Source: CAD feature listing. Evaluate the final solid. Frame: model axes, mm. Face numbers are marked on the shaded views. A direction names the side the tool comes from. Round coordinates to 2 decimals unless told otherwise and drop trailing zeros. Loops run counter-clockwise (first coordinate to the right, second up) from the corner with the lowest first, then second, coordinate; pieces in that order, holes last. Notation, with made-up numbers: (62, -29.5) -> (111, -29.5) arc R16 cw to (111, -18.5) -> close; hole circle Ø11 at (55.25, -3). An arc over 180 degrees is marked (long way). Put each result on its own line as item: value. Start each with the question number.
1. Cut plane D-D (x = -4). Return the cut outline in (y, z), then the cut area to 3 significant figures.
2. Contact query for flat-ended pins moving along their axis: pin 1 (1.6 mm diameter, centred on x = 3.45, y = -84.2, fed in from -Z); pin 2 (3 mm diameter, centred on y = -9.5, z = 4.25, fed in from +X); pin 3 (4 mm diameter, centred on x = 4.5, z = -7, fed in from -Y). Output: stop coordinate, or through.
3. Cut plane C-C (y = -60.5). Return the cut outline in (x, z).
4. Set-up query: the marked faces 1 and 2. Return all of +Z, -Z, +X, -X, +Y, -Y with unobstructed straight access to the full face (end or side cutting, diameter ignored); none if empty.
5. Material intervals for L1, parallel to X at y = -84.2, z = 2; L2, parallel to Y at x = 3.45, z = 1.75; L3, parallel to X at y = -101.05, z = -5, sorted ascending.
6. Cut plane A-A (y = -97). Return the cut outline in (x, z), then the cut area to 3 significant figures.
7. Cut plane B-B (z = -1.5). Return the cut outline in (x, y), then the cut area to 3 significant figures.
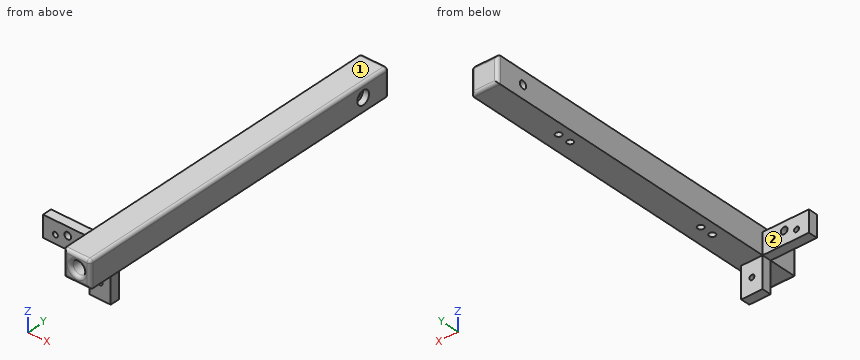
```python
from build123d import *

# Parameters (mm, degrees)
SKETCH1_W                      = 8.5
SKETCH1_H                      = 111.5
BOSS_EXTRUDE5_DEPTH            = 8.5
M5X0_8_TAPPED_HOLE2_D          = 4.2
M5X0_8_TAPPED_HOLE2_DEPTH      = 20
M5X0_8_TAPPED_HOLE2_TIP        = 1.2618073
SKETCH35_W                     = 8.5
SKETCH35_H                     = 3
BOSS_EXTRUDE6_DEPTH            = 15
F_2_2_2_2_DIAMETER_HOLE1_D     = 2.2
F_2_2_2_2_DIAMETER_HOLE1_DEPTH = 13
M2X0_4_TAPPED_HOLE5_D          = 1.6
M2X0_4_TAPPED_HOLE5_DEPTH      = 3
SKETCH40_W                     = 8.5
SKETCH40_H                     = 3
BOSS_EXTRUDE7_DEPTH            = 10
M2X0_4_TAPPED_HOLE4_D          = 1.6
M2X0_4_TAPPED_HOLE4_DEPTH      = 3
FILLET1_R                      = 1
M2X0_4_TAPPED_HOLE3_D          = 2
M2X0_4_TAPPED_HOLE3_DEPTH      = 5.2
M2X0_4_TAPPED_HOLE3_TIP        = 0.600860619
SKETCH49_W                     = 1.6
SKETCH49_H                     = 10
SKETCH49_W_2                   = 15
SKETCH49_H_2                   = 1.6
CUT_EXTRUDE1_DEPTH             = 10


with BuildPart() as part:
    # Sketch1 → Boss-Extrude5 (new body)
    with BuildSketch(Plane.XY):
        with Locations((4.25, -55.75)):
            Rectangle(SKETCH1_W, SKETCH1_H)
    extrude(amount=BOSS_EXTRUDE5_DEPTH)

    # M5x0.8 Tapped Hole2
    with Locations(Plane(origin=(0, -111.5, 0), x_dir=(-1, 0, 0), z_dir=(0, -1, 0))):
        with Locations((-4.25, -4.25)):
            Hole(M5X0_8_TAPPED_HOLE2_D / 2, depth=M5X0_8_TAPPED_HOLE2_DEPTH)
            with Locations((0, 0, -(M5X0_8_TAPPED_HOLE2_DEPTH + M5X0_8_TAPPED_HOLE2_TIP / 2))):  # 118° drill point
                Cone(0, M5X0_8_TAPPED_HOLE2_D / 2, M5X0_8_TAPPED_HOLE2_TIP, mode=Mode.SUBTRACT)

    # Sketch35 → Boss-Extrude6 (add)
    with BuildSketch(Plane.ZY):
        with Locations((4.25, -100.5)):
            Rectangle(SKETCH35_W, SKETCH35_H)
    extrude(amount=BOSS_EXTRUDE6_DEPTH)

    # Ø2.2 (2.2) Diameter Hole1
    with Locations(Plane(origin=(0, -99, 0), x_dir=(1, 0, 0), z_dir=(0, 1, 0))):
        with Locations((-7, -4.2)):
            Hole(F_2_2_2_2_DIAMETER_HOLE1_D / 2, depth=F_2_2_2_2_DIAMETER_HOLE1_DEPTH)

    # M2x0.4 Tapped Hole5
    with Locations(Plane(origin=(0, -99, 0), x_dir=(1, 0, 0), z_dir=(0, 1, 0))):
        with Locations((-11, -2.75)):
            Hole(M2X0_4_TAPPED_HOLE5_D / 2, depth=M2X0_4_TAPPED_HOLE5_DEPTH)

    # Sketch40 → Boss-Extrude7 (add)
    with BuildSketch(Plane(origin=(0, 0, 0), x_dir=(-1, 0, 0), z_dir=(0, 0, -1))):
        with Locations((-4.25, -100.5)):
            Rectangle(SKETCH40_W, SKETCH40_H)
    extrude(amount=BOSS_EXTRUDE7_DEPTH)

    # M2x0.4 Tapped Hole4
    with Locations(Plane(origin=(0, -99, 0), x_dir=(1, 0, 0), z_dir=(0, 1, 0))):
        with Locations((3.45, 5)):
            Hole(M2X0_4_TAPPED_HOLE4_D / 2, depth=M2X0_4_TAPPED_HOLE4_DEPTH)

    # Sketch45 → CBORE for M2 Socket Head Cap Screw1 (revolve, cut)
    with BuildSketch(Plane(origin=(8.5, -9.5, 4.25), x_dir=(0, 0, -1), z_dir=(0, 1, 0))):
        Polygon((0, 0), (0, 23.500025), (1.2, 23.500025), (1.2, 2.025), (1.225, 2), (2.2, 2), (2.2, 0), align=None)
    revolve(axis=Axis((14.85, -9.5, 4.25), (-1, 0, 0)), mode=Mode.SUBTRACT)

    # Fillet1
    fillet1_edges = [part.edges().sort_by_distance(p)[0] for p in [
        (4.25, 0, 8.5),
        (2.15, -111.5, 4.25),
        (8.5, -55.75, 8.5),
        (4.25, 0, 0),
        (4.25, -111.5, 0),
        (4.25, -111.5, 8.5),
        (8.5, 0, 4.25),
        (0, 0, 4.25),
        (0, -111.5, 4.25),
        (8.5, -111.5, 4.25),
    ]]
    fillet(fillet1_edges, radius=FILLET1_R)

    # M2x0.4 Tapped Hole3
    with Locations(Plane(origin=(0, 0, 0), x_dir=(-1, 0, 0), z_dir=(0, 0, -1))):
        with Locations((-3.45, -26.8), (-3.45, -84.2), (-3.45, -31.1), (-3.45, -79.9)):
            Hole(M2X0_4_TAPPED_HOLE3_D / 2, depth=M2X0_4_TAPPED_HOLE3_DEPTH)
            with Locations((0, 0, -(M2X0_4_TAPPED_HOLE3_DEPTH + M2X0_4_TAPPED_HOLE3_TIP / 2))):  # 118° drill point
                Cone(0, M2X0_4_TAPPED_HOLE3_D / 2, M2X0_4_TAPPED_HOLE3_TIP, mode=Mode.SUBTRACT)

    # Sketch49 → Cut-Extrude1 (cut)
    with BuildSketch(Plane(origin=(0, -99, 0), x_dir=(1, 0, 0), z_dir=(0, 1, 0))):
        with Locations((7.7, 5)):
            Rectangle(SKETCH49_W, SKETCH49_H)
        with Locations((-7.5, -7.7)):
            Rectangle(SKETCH49_W_2, SKETCH49_H_2)
    extrude(amount=-CUT_EXTRUDE1_DEPTH, mode=Mode.SUBTRACT)


solid = part.part
```
Solution:
1. outline: (-102, 0) -> (-99, 0) -> (-99, 6.9) -> (-102, 6.9) -> close
1. area: 20.7 mm^2
2. pin 1: stops at z = 5.32
2. pin 2: stops at x = 6.5
2. pin 3: stops at y = -102
3. outline: (0, 0) -> (8.5, 0) -> (8.5, 7.5) arc R1 ccw to (7.5, 8.5) -> (0, 8.5) -> close
4. face 1: +Z, +X, -X, +Y, -Y
4. face 2: +Z, -Z, -X, +Y
5. L1: x = 0 to 2.45, 4.45 to 8.5
5. L2: y = -111.38 to -85.2, -83.2 to -80.9, -78.9 to -32.1, -30.1 to -27.8, -25.8 to 0
5. L3: x = 0 to 2.65, 4.25 to 6.9
6. outline: (0, 0) -> (8.5, 0) -> (8.5, 7.5) arc R1 ccw to (7.5, 8.5) -> (0, 8.5) -> close; hole circle Ø4.2 at (4.25, 4.25)
6. area: 58.2 mm^2
7. outline: (0, -102) -> (6.9, -102) -> (6.9, -99) -> (0, -99) -> close
7. area: 20.7 mm^2
